from build123d import *

# Parameters (mm, degrees)
ESBO_O2_W             = 1.2
ESBO_O2_H             = 1.2
CORTE_EXTRUS_O1_DEPTH = 1


with BuildPart() as part:
    # Esboço1 → Revolução1 (revolve)
    with BuildSketch(Plane(origin=(0, 0, 0), x_dir=(0, 1, 0), z_dir=(0, 0, 1))):
        Polygon((0, 5.5), (-2.5, 5.5), (-2.5, -2.5), (-3.75, -2.5), (-3.75, -3.560606061), (-3.75, -6), (-2, -6), (-2, -5.5), (0, -5.5), align=None)
    revolve(axis=Axis((-5.5, 0, 0), (1, 0, 0)))

    # Esboço2 → Corte-extrusão1 (cut)
    with BuildSketch(Plane.ZY.offset(5.5)):
        Polygon((-0.66395281, -1.15), (1.327905619, 0), (-0.66395281, 1.15), align=None)
        with Locations((-1.26395281, 0)):
            Rectangle(ESBO_O2_W, ESBO_O2_H)
    extrude(amount=-CORTE_EXTRUS_O1_DEPTH, mode=Mode.SUBTRACT)


solid = part.part
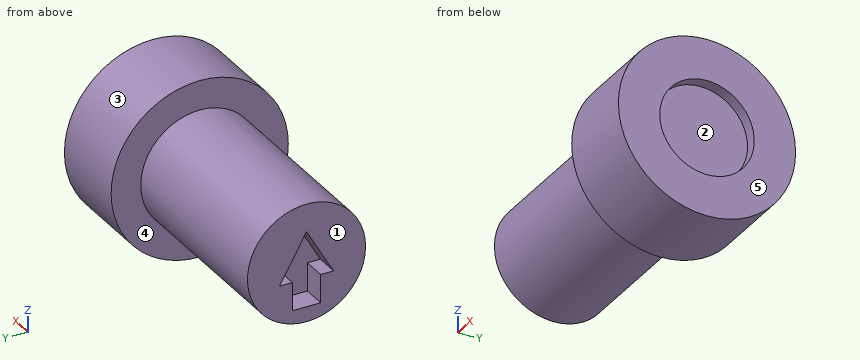
Here's how the part is built. I have some questions about the finished solid (model axes, mm). Face numbers are marked on the shaded views. A direction names the side the tool comes from. Coordinates: 2 decimals unless noted, no trailing zeros. Loops run counter-clockwise (first coordinate to the right, second up) from the corner with the lowest first, then second, coordinate; pieces in that order, holes last. Notation, with made-up numbers: (44, 62.5) -> (57, 62.5) arc R23 cw to (57, 97.5) -> close; hole circle Ø8 at (41, -24). An arc over 180 degrees is marked (long way). Use one line per item in the form item = value. Start each with the question number.
(1) Will these pins go through, and if not, where does the flat tip stop? pin 1 (0.8 mm diameter, centred on x = -5, z = -1, fed in from +Y); pin 2 (0.5 mm diameter, centred on x = -5, y = 0, fed in from +Z); pin 3 (1 mm diameter, centred on y = -2.5, z = -2.5, fed in from -X).
(2) We'd pull the mould along Y, two halves only. Please class the marked faces 1, 2 and 3: pulls with the +Y half, pulls with the -Y half, needs draft (parallel to the pull), parting line crosses it, or undercut.
(3) If we section it at B-B (y = 1): Please give me the cut outline in (x, z), then the cut area to 3 significant figures.
(4) Please list where these lines run through material, in increasing order: line 1 along Z through (x, y) = (5.75, 0); line 2 along Z through (x, y) = (-2.75, 1.5).
(5) On a 3-axis mill with a long thin cutter (end or side, diameter ignored), from which of +Z, -Z, +X, -X, +Y, -Y can I reach the whole of each face in a straight line? I mean the marked faces 4 and 5. Say none if no direction works.
(6) If we section it at C-C (z = 0): Please give me the cut outline in (x, y), then the cut area to 3 significant figures.
(7) If we section it at D-D (x = 4.75): Please give me the cut outline in (y, z), then the cut area to 3 significant figures.
(8) If we section it at A-A (x = -0.25): Please give me the cut outline in (y, z).
Verdict:
q1.pin_1 = 2.43
q1.pin_2 = 2.5
q1.pin_3 = 2.5
q2.face_1 = needs draft
q2.face_2 = undercut
q2.face_3 = parting line crosses it
q3.outline = (-5.5, -2.29) -> (2.5, -2.29) -> (2.5, -3.61) -> (6, -3.61) -> (6, -1.73) -> (5.5, -1.73) -> (5.5, 1.73) -> (6, 1.73) -> (6, 3.61) -> (2.5, 3.61) -> (2.5, 2.29) -> (-5.5, 2.29) -> (-5.5, -0.4) -> (-4.5, -0.4) -> (-4.5, -0.66) -> (-5.5, -0.66) -> close
q3.area = 60.0 mm²
q4.line_1 = -3.75 to -2, 2 to 3.75
q4.line_2 = -2 to 2
q5.face_4 = -X
q5.face_5 = +Z, -Z, +X, +Y, -Y
q6.outline = (-5.5, -2.5) -> (2.5, -2.5) -> (2.5, -3.75) -> (6, -3.75) -> (6, -2) -> (5.5, -2) -> (5.5, 2) -> (6, 2) -> (6, 3.75) -> (2.5, 3.75) -> (2.5, 2.5) -> (-5.5, 2.5) -> (-5.5, 0.77) -> (-4.5, 0.77) -> (-4.5, -0.77) -> (-5.5, -0.77) -> close
q6.area = 62.7 mm²
q7.outline = circle Ø7.5 at (0, 0)
q7.area = 44.2 mm²
q8.outline = circle Ø5 at (0, 0)
